Geometry: final body of the model. Coordinates: model frame, mm. A direction names the side the tool comes from. Round coordinates to 2 decimals unless told otherwise and drop trailing zeros. Loops run counter-clockwise (first coordinate to the right, second up) from the corner with the lowest first, then second, coordinate; pieces in that order, holes last. Notation, with made-up numbers: M 59,72 L 89,72 A20 ccw 89,99 Z; hole C -8,-19 d5. An arc over 180 degrees is marked long. Write each question's results on one line, items separated by ' | '.
```python
from build123d import *

# Parameters (mm, degrees)
F1_DEPTH = 19.4
F2_DEPTH = 1.2
F3_W     = 25
F3_H     = 7.2
F4_DEPTH = 1.2
F5_W     = 16.95
F5_H     = 7.1
F6_DEPTH = 9
F7_W     = 2.4
F7_H     = 1.2
F8_ANGLE = 180


with BuildPart() as f1:
    # F0 (on Right) → F1 (new body)
    with BuildSketch(Plane.YZ):
        Polygon((-8.668413, 6.839403), (-18.668413, 6.839403), (-18.668413, -2.360597), (-8.668413, -2.360597), (-8.668413, -1.360597), (-8.668413, 2.239403), (-8.668413, 5.839403), align=None)
    extrude(amount=F1_DEPTH)

    # F0 (on Right) → F2 (join)
    with BuildSketch(Plane.YZ):
        Polygon((-8.668413, 6.839403), (-18.668413, 6.839403), (-18.668413, -2.360597), (-8.668413, -2.360597), (-8.668413, -1.360597), (-8.668413, 2.239403), (-8.668413, 5.839403), align=None)
        Polygon((16.331587, 5.839403), (-8.668413, 5.839403), (-8.668413, 2.239403), (-8.668413, -1.360597), (16.331587, -1.360597), align=None)
        with BuildLine():
            ThreePointArc((11.531587, 3.439403), (12.731587, 2.239403), (11.531587, 1.039403))
            Line((11.531587, 1.039403), (0.931587, 1.039403))
            ThreePointArc((0.931587, 1.039403), (-0.268413, 2.239403), (0.931587, 3.439403))
            Line((0.931587, 3.439403), (11.531587, 3.439403))
        make_face(mode=Mode.SUBTRACT)
    extrude(amount=F2_DEPTH)

    # F3 (on face) → F4 (join)
    with BuildSketch(Plane.YZ.offset(19.4)):
        with Locations((3.831587, 2.239403)):
            Rectangle(F3_W, F3_H)
        with BuildLine():
            ThreePointArc((11.531587, 3.439403), (12.731587, 2.239403), (11.531587, 1.039403))
            Line((11.531587, 1.039403), (0.931587, 1.039403))
            ThreePointArc((0.931587, 1.039403), (-0.268413, 2.239403), (0.931587, 3.439403))
            Line((0.931587, 3.439403), (11.531587, 3.439403))
        make_face(mode=Mode.SUBTRACT)
    extrude(amount=-F4_DEPTH)

    # F5 (on face) → F6 (cut)
    with BuildSketch(Plane(origin=(0, -8.668413, 0), x_dir=(-1, 0, 0), z_dir=(0, 1, 0))):
        with Locations((-9.725, 2.239403)):
            Rectangle(F5_W, F5_H)
    extrude(amount=-F6_DEPTH, mode=Mode.SUBTRACT)

    # F7 (on face) → F8 (revolve)
    with BuildSketch(Plane.YZ.offset(19.4)):
        with Locations((-11.550809, 2.537114)):
            Rectangle(F7_W, F7_H)
    revolve(axis=Axis((19.4, -13.350809, 2.537114), (0, 0, -1)), revolution_arc=F8_ANGLE)


solid = f1.part
```
1. Access query for faces 5 (the face through (1, 4, -1.361)), 6 (the face through (19, 6, 1.039)), 7 (the face through (1, 4, 5.839)), 8 (the face through (21, -13, 3.137)), 9 (the face through (18.2, -1, 2)). Directions: +Z, -Z, +X, -X, +Y, -Y. A direction counts if a zero-diameter tool reaches every point of the face in a straight line with its end or side. Return the directions, or none.
Answer key:
face 5: -Z, +X, -X, +Y | face 6: +X, -X | face 7: +Z, +X, -X, +Y | face 8: +Z, +X, +Y, -Y | face 9: +Y
2. Pin query (flat end, axial travel): P1, Ø0.6, axis at x = 0.5, y = 8, coming from the +Z side; P2, Ø3, axis at y = 5, z = 0.5, coming from the +X side; P3, Ø1.3, axis at x = 19, y = 3.5, coming from the -Z side. Return the tip coordinate at first contact, or that it passes through.
Answer key:
P1: stops at z = 5.84 | P2: stops at x = 19.4 | P3: stops at z = -1.36
3. Ray query, probe 1 along X at (y, z) = (-6.5, 1); probe 2 along Z at (x, y) = (5, -10); probe 3 along Y at (x, z) = (6, -0.75). Return the intervals inside material, ascending.
Answer key:
probe 1: x = 0 to 1.2, 18.2 to 19.4 | probe 2: z = -2.36 to -1.31, 5.79 to 6.84 | probe 3: y = -18.67 to -17.67
4. Draft query along Y for faces 1 (the face through (19, 16.332, 2)), 2 (the face through (22.4, -13.3, 2.5)), 3 (the face through (0, -5, 2)), 4 (the face through (0.59, -0.27, 2.21)). Return one class per face: pulls with the +Y half, pulls with the -Y half, needs draft (parallel to the pull), parting line crosses it, or undercut.
Answer key:
face 1: pulls with the +Y half | face 2: parting line crosses it | face 3: needs draft | face 4: undercut
5. Section C-C (x = 7.75). Output: boundary loops of the cut face in (y, z).
Answer key:
outline: M -18.67,-2.36 L -8.67,-2.36 L -8.67,-1.31 L -17.67,-1.31 L -17.67,5.79 L -8.67,5.79 L -8.67,6.84 L -18.67,6.84 Z
6. Section A-A (y = -5). Output: boundary loops of the cut face in (x, z), then the cut area to 3 significant figures.
Answer key:
outline: M 0,-1.36 L 1.2,-1.36 L 1.2,5.84 L 0,5.84 Z; M 18.2,-1.36 L 19.4,-1.36 L 19.4,5.84 L 18.2,5.84 Z | area: 17.3 mm²
7. Section B-B (y = 11). Output: boundary loops of the cut face in (x, z).
Answer key:
outline: M 0,-1.36 L 1.2,-1.36 L 1.2,1.04 L 0,1.04 Z; M 0,3.44 L 1.2,3.44 L 1.2,5.84 L 0,5.84 Z; M 18.2,-1.36 L 19.4,-1.36 L 19.4,1.04 L 18.2,1.04 Z; M 18.2,3.44 L 19.4,3.44 L 19.4,5.84 L 18.2,5.84 Z
8. Section D-D (z = 0.5). Output: boundary loops of the cut face in (x, y), then the cut area to 3 significant figures.
Answer key:
outline: M 0,-18.67 L 19.4,-18.67 L 19.4,16.33 L 18.2,16.33 L 18.2,-17.67 L 1.25,-17.67 L 1.25,-8.67 L 1.2,-8.67 L 1.2,16.33 L 0,16.33 Z | area: 101 mm²
